```python
from build123d import *

# Parameters (mm, degrees)
RESSALTO_EXTRUS_O1_DEPTH = 28.35
ESBO_O2_R                = 4.25
CORTE_EXTRUS_O1_DEPTH    = 26
ESBO_O3_W                = 36.7
ESBO_O3_H                = 41.8
RESSALTO_EXTRUS_O2_DEPTH = 14.75
ESBO_O5_W                = 30.5
ESBO_O5_H                = 20.5
CORTE_EXTRUS_O2_DEPTH    = 13.2
CORTE_EXTRUS_O3_DEPTH    = 69.850889609
ESBO_O7_W                = 5
ESBO_O7_H                = 16.7
CORTE_EXTRUS_O4_DEPTH    = 6.5
FILETE1_R                = 2.5
ESBO_O8_W                = 8.5
ESBO_O8_H                = 3.5
CORTE_EXTRUS_O5_DEPTH    = 14
ESBO_O9_W                = 3.2
ESBO_O9_H                = 3.2
RESSALTO_EXTRUS_O3_DEPTH = 2


with BuildPart() as part:
    # Esboço1 → Ressalto-extrusão1 (new body)
    with BuildSketch(Plane.XY):
        with BuildLine():
            Line((14.1, -8.525), (14.1, 22.625))
            Line((14.1, 22.625), (-14.1, 22.625))
            Line((-14.1, 22.625), (-14.1, -8.525))
            ThreePointArc((-14.1, -8.525), (0, -22.625), (14.1, -8.525))
        make_face()
    extrude(amount=RESSALTO_EXTRUS_O1_DEPTH)

    # Esboço2 → Corte-extrusão1 (cut)
    with BuildSketch(Plane(origin=(0, 0, 0), x_dir=(-1, 0, 0), z_dir=(0, 0, -1))):
        with Locations((0, -13.375)):
            Circle(ESBO_O2_R)
    extrude(amount=-CORTE_EXTRUS_O1_DEPTH, mode=Mode.SUBTRACT)

    # Esboço3 → Ressalto-extrusão2 (add)
    with BuildSketch(Plane(origin=(0, 22.625, 0), x_dir=(1, 0, 0), z_dir=(0, 1, 0))):
        with Locations((0, -7.45)):
            Rectangle(ESBO_O3_W, ESBO_O3_H)
    extrude(amount=RESSALTO_EXTRUS_O2_DEPTH)

    # Esboço5 → Corte-extrusão2 (cut)
    with BuildSketch(Plane(origin=(0, 37.375, 0), x_dir=(1, 0, 0), z_dir=(0, 1, 0))):
        with Locations((0, -13.5)):
            Rectangle(ESBO_O5_W, ESBO_O5_H)
    extrude(amount=-CORTE_EXTRUS_O2_DEPTH, mode=Mode.SUBTRACT)

    # Esboço6 → Corte-extrusão3 (cut, through all)
    with BuildSketch(Plane(origin=(0, 37.375, 0), x_dir=(1, 0, 0), z_dir=(0, 1, 0))):
        with BuildLine():
            Line((-2, 13.45), (-2, 6.30835312))
            ThreePointArc((-2, 6.30835312), (0, 4.30835312), (2, 6.30835312))
            Line((2, 6.30835312), (2, 13.45))
            Line((2, 13.45), (-2, 13.45))
        make_face()
    extrude(amount=-CORTE_EXTRUS_O3_DEPTH, mode=Mode.SUBTRACT)

    # Esboço7 → Corte-extrusão4 (cut)
    with BuildSketch(Plane(origin=(0, 37.375, 0), x_dir=(1, 0, 0), z_dir=(0, 1, 0))):
        with Locations((-9.55, 5.1)):
            Rectangle(ESBO_O7_W, ESBO_O7_H)
        with Locations((9.55, 5.1)):
            Rectangle(ESBO_O7_W, ESBO_O7_H)
    extrude(amount=-CORTE_EXTRUS_O4_DEPTH, mode=Mode.SUBTRACT)

    # Filete1
    filete1_edges = [part.edges().sort_by_distance(p)[0] for p in [
        (-12.05, 30.875, -5.1),
        (-7.05, 30.875, -5.1),
        (7.05, 30.875, -5.1),
        (12.05, 30.875, -5.1),
    ]]
    fillet(filete1_edges, radius=FILETE1_R - 0.0001)  # a hair under: the kernel refuses the full size

    # Esboço8 → Corte-extrusão5 (cut)
    with BuildSketch(Plane(origin=(0, 0, -13.45), x_dir=(-1, 0, 0), z_dir=(0, 0, -1))):
        with Locations((0.04245602, 30)):
            Rectangle(ESBO_O8_W, ESBO_O8_H)
    extrude(amount=-CORTE_EXTRUS_O5_DEPTH, mode=Mode.SUBTRACT)

    # Esboço9 → Ressalto-extrusão3 (add)
    with BuildSketch(Plane(origin=(0, 37.375, 0), x_dir=(1, 0, 0), z_dir=(0, 1, 0))):
        with Locations((-13.65, -1.65)):
            Rectangle(ESBO_O9_W, ESBO_O9_H)
        with Locations((13.65, -1.65)):
            Rectangle(ESBO_O9_W, ESBO_O9_H)
    extrude(amount=RESSALTO_EXTRUS_O3_DEPTH)


solid = part.part
```
For this review, take the finished solid that the model builds, in its own axes (mm). A direction names the side the tool comes from. Round coordinates to 2 decimals unless told otherwise and drop trailing zeros. Order: outer loops, then holes, each group sorted by start corner. A loop starts at its lowest first (then second) coordinate and runs counter-clockwise, first axis right, second up.
Q1. Insertion check: P1, Ø6, axis at x = -5, z = 11.5, coming from the +Y side (3 decimals); P2, Ø14, axis at x = 0, y = -2.5, coming from the -Z side; P3, Ø9.5, axis at x = -1.5, z = -6.5, coming from the +Y side (3 decimals). Each pin has a flat end and moves straight along its axis. Give the tip position at first contact, or say it passes through.
Findings below:
P1: stops at y = 24.175
P2: stops at z = 0
P3: stops at y = 37.375
Q2. We need section B-B, the plane z = 17.5. Give the boundary of the cut face in (x, y) (3 decimals), plus the area to 3 significant figures.
Findings below:
outline: (-18.35, 22.625) - (-14.1, 22.625) - (-14.1, -8.525) arc R14.1 ccw to (14.1, -8.525) - (14.1, 22.625) - (18.35, 22.625) - (18.35, 37.375) - (15.25, 37.375) - (15.25, 24.175) - (-15.25, 24.175) - (-15.25, 37.375) - (-18.35, 37.375) - close; hole circle Ø8.5 at (0, -13.375)
area: 1,270 mm2
Q3. Wall thickness on line 1 (Y direction, x = 0, z = 6.5) (3 decimals); line 2 (X direction, y = 30, z = 12.5); line 3 (Z direction, x = -9.5, y = 8): over which ranges is each line inside the solid? List them lowest first.
Findings below:
line 1: y = -22.625 to -17.625, -9.125 to 24.175
line 2: x = -18.35 to -15.25, 15.25 to 18.35
line 3: z = 0 to 28.35
Q4. Machinability: for faces 4 (the cylindrical face through (11.34, 31.63, -5.22)), 5 (the flat face through (0, 28.25, -3)), 6 (the flat face through (-14.1, 7, 14)), 7 (the flat face through (14, 38, 0.05)), which of the approach directions +Z, -Z, +X, -X, +Y, -Y give a long, thin tool a straight path to every point of the face, cutting with its end or side? Answer none if there is none.
Findings below:
face 4: -Z, +Y
face 5: -Z
face 6: +Z, -Z, -X, -Y
face 7: -Z, +X, -X, +Y
Q5. We need section C-C, the plane y = -2. Give the boundary of the cut face in (x, z).
Findings below:
outline: (-14.1, 0) - (14.1, 0) - (14.1, 28.35) - (-14.1, 28.35) - close
Q6. Mouldability with a two-part tool opening along X and no side actions: class faces 1 (the flat face through (12.05, 36, -5)), 2 (the flat face through (-10, 30, -13.45)), 3 (the flat face through (15.25, 38, 2)) as pulls with the +X half, pulls with the -X half, needs draft (parallel to the pull), parting line crosses it, or undercut.
Findings below:
face 1: undercut
face 2: needs draft
face 3: pulls with the +X half
Q7. We need section D-D, the plane x = -8.5. Give the boundary of the cut face in (y, z) (3 decimals).
Findings below:
outline: (-19.775, 0) - (22.625, 0) - (22.625, -13.45) - (31.106, -13.45) - (31.106, 3.25) - (24.175, 3.25) - (24.175, 23.75) - (37.375, 23.75) - (37.375, 28.35) - (-19.775, 28.35) - close
Q8. We need section A-A, the plane x = 0. Give the boundary of the cut face in (y, z) (3 decimals), plus the area to 3 significant figures.
Findings below:
outline: (-22.625, 0) - (-17.625, 0) - (-17.625, 26) - (-9.125, 26) - (-9.125, 0) - (22.625, 0) - (22.625, -4.308) - (28.25, -4.308) - (28.25, 0.55) - (31.75, 0.55) - (31.75, -4.308) - (37.375, -4.308) - (37.375, 3.25) - (24.175, 3.25) - (24.175, 23.75) - (37.375, 23.75) - (37.375, 28.35) - (-22.625, 28.35) - close
area: 1,260 mm2
